```python
from build123d import *

# Parameters (mm, degrees)
BOSS_EXTRUDE1_DEPTH  = 8
M5_CLEARANCE_HOLE1_D = 5.3
FILLET1_R            = 5


with BuildPart() as part:
    # Sketch1 → Boss-Extrude1 (new body)
    with BuildSketch(Plane.XY):
        Polygon((-98, -30), (98, -30), (98, 0), (38, 170), (-38, 170), (-98, 0), align=None)
    extrude(amount=BOSS_EXTRUDE1_DEPTH)

    # M5 Clearance Hole1 (through all)
    with Locations(Plane.XY.offset(8)):
        with Locations((-23, 150), (-23, 67.5), (-23, -15), (23, -15), (23, 150), (23, 67.5), (-83, -15), (83, -15)):
            Hole(M5_CLEARANCE_HOLE1_D / 2)

    # Fillet1
    fillet1_edges = [part.edges().sort_by_distance(p)[0] for p in [
        (-98, 0, 4),
        (-38, 170, 4),
        (38, 170, 4),
        (98, 0, 4),
        (98, -30, 4),
        (-98, -30, 4),
    ]]
    fillet(fillet1_edges, radius=FILLET1_R)


solid = part.part
```
Read the model definition and answer for the solid it produces. Units are mm, in the model's axes. Round coordinates to 2 decimals unless told otherwise and drop trailing zeros. Loops run counter-clockwise (first coordinate to the right, second up) from the corner with the lowest first, then second, coordinate; pieces in that order, holes last. Notation, with made-up numbers: (-33, 0.25) -> (25, 0.25) arc R21 ccw to (25, 38.25) -> close; hole circle Ø10 at (-16.75, 3.25). An arc over 180 degrees is marked (long way). One line per item, written item: value.
1) A cutting plane is placed at B-B (x = 23). Determine the outline of the cut face in (y, z).
Answer list:
outline: (-30, 0) -> (-17.65, 0) -> (-17.65, 8) -> (-30, 8) -> close; (-12.35, 0) -> (64.85, 0) -> (64.85, 8) -> (-12.35, 8) -> close; (70.15, 0) -> (147.35, 0) -> (147.35, 8) -> (70.15, 8) -> close; (152.65, 0) -> (170, 0) -> (170, 8) -> (152.65, 8) -> close
2) Consider L1, parallel to Y at x = 23, z = 1.75; L2, parallel to Y at x = 22, z = 0.5; L3, parallel to X at y = 150, z = 6.25. Determine where each line is inside the solid, lowest interval first. Write a range as [from, to].
Answer list:
L1: y = [-30, -17.65], [-12.35, 64.85], [70.15, 147.35], [152.65, 170]
L2: y = [-30, -17.45], [-12.55, 65.05], [69.95, 147.55], [152.45, 170]
L3: x = [-45.06, -25.65], [-20.35, 20.35], [25.65, 45.06]
3) A cutting plane is placed at D-D (y = 67.5). Determine the outline of the cut face in (x, z), and give its area (3 significant figures).
Answer list:
outline: (-74.18, 0) -> (-25.65, 0) -> (-25.65, 8) -> (-74.18, 8) -> close; (-20.35, 0) -> (20.35, 0) -> (20.35, 8) -> (-20.35, 8) -> close; (25.65, 0) -> (74.18, 0) -> (74.18, 8) -> (25.65, 8) -> close
area: 1,100 mm²
4) A cutting plane is placed at C-C (x = 83). Determine the outline of the cut face in (y, z), and give its area (3 significant figures).
Answer list:
outline: (-30, 0) -> (-17.65, 0) -> (-17.65, 8) -> (-30, 8) -> close; (-12.35, 0) -> (42.5, 0) -> (42.5, 8) -> (-12.35, 8) -> close
area: 538 mm²
5) The mould has two halves that part along Y. Classify faces 1 (the face through (-96, -29, 4)), 2 (the face through (98, -13, 4)), 3 (the face through (21.777, -17.351, 3.944)), 4 (the face through (68.856, 82.575, 3.944)): pulls with the +Y half, pulls with the -Y half, needs draft (parallel to the pull), parting line crosses it, or undercut.
Answer list:
face 1: pulls with the -Y half
face 2: needs draft
face 3: undercut
face 4: pulls with the +Y half
6) Flat-ended cylindrical pins translate along their axes: P1, Ø4, axis at y = 6, z = 6.5, coming from the -X side; P2, Ø2, axis at y = 8, z = 1, coming from the -X side; P3, Ø3, axis at y = 102, z = 3.5, coming from the +X side. Find the tip coordinate at first contact, or state that the pin passes through.
Answer list:
P1: stops at x = -96.59
P2: stops at x = -95.53
P3: stops at x = 62.53
7) A cutting plane is placed at A-A (z = 3.25). Give the number of separate pieces and of enclosed holes in the cut face, and give its area (3 significant figures).
Answer list:
separate pieces: 1
enclosed holes: 8
area: 28,800 mm²
